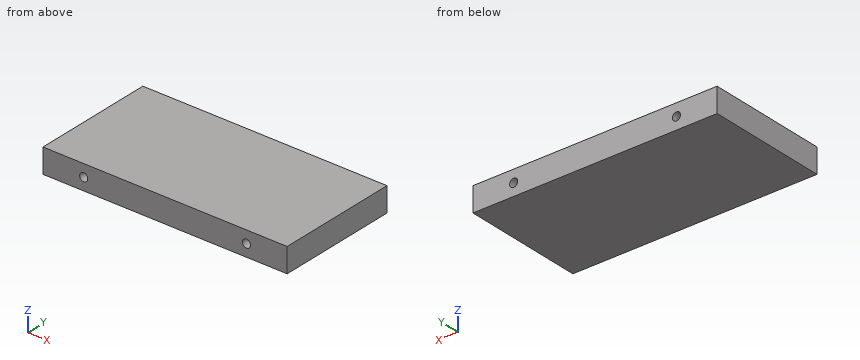
Autodesk Inventor part; units mm, degrees
ref_plane "YZ Plane" through (0, 0, 0) normal (1, 0, 0) x (0, 1, 0)
ref_plane "XZ Plane" through (0, 0, 0) normal (0, 1, 0) x (-1, 0, 0)
ref_plane "XY Plane" through (0, 0, 0) normal (0, 0, 1) x (1, 0, 0)
sketch "Skizze1" plane through (0, 0, 0) normal (0, 1, 0) x (-1, 0, 0)
  line L0 (0, 0) -> (60, 0)
  line L1 (60, 0) -> (60, -6)
  line L2 (60, -6) -> (0, -6)
  line L3 (0, -6) -> (0, 0)
  dimension "d0" = 60
  dimension "d1" = 6
extrude "Extrusion1" add sketch "Skizze1" along normal blind 30
sketch "m" plane through (0, 0, 0) normal (0, -1, 0) x (1, 0, 0)
  line L0 (0, -6) -> (0, 0)
  line L1 (-60, -6) -> (0, -6)
  point P0 (-10, -3)
  point P1 (-50, -3)
  dimension "d4" = 40
  dimension "d5" = 10
  dimension "d6" = 3
hole "Bohrung1" at (-10, 0, -3) at (-50, 0, -3) direction (0, 1, 0) diameter 2 depth 10 tip angle 118
sketch "Skizze3" plane through (0, 30, 0) normal (0, 1, 0) x (1, 0, 0)
  point P0 (0, 0)
  point P1 (-10, 3)
  point P2 (-50, 3)
hole "Bohrung2" at (-10, 30, -3) at (-50, 30, -3) direction (0, -1, 0) diameter 2 depth 10 tip angle 118
properties part number "AkkuHaltSeitenWand"
Geometry: final body of the model. Coordinates: model frame, mm. Give positions to 0.01 mm unless a question says otherwise; leave off trailing zeros. Loops run counter-clockwise (first coordinate to the right, second up) from the corner with the lowest first, then second, coordinate; pieces in that order, holes last. Notation, with made-up numbers: M 23,19 L 57,19 A9 ccw 57,34 Z; hole C 26,41 d6. An arc over 180 degrees is marked long. Put each result on its own line as item: value. Start each with the question number.
1) Cut plane A-A (y = 5.25). Output: boundary loops of the cut face in (x, z), then the cut area to 3 significant figures.
2) Contact query for flat-ended pins moving along their axis: pin 1 (1.2 mm diameter, centred on x = -10, z = -3, fed in from +Y); pin 2 (1.5 mm diameter, centred on x = -26.5, z = -5, fed in from -Y); pin 3 (1.8 mm diameter, centred on x = -10, z = -3, fed in from +Y). Output: stop coordinate, or through.
3) Ray query, line 1 along X through (y, z) = (4.25, -3); line 2 along Z through (x, y) = (-10, 26.5). Return the intervals inside material, ascending.
Verdict:
1. outline: M -60,-6 L 0,-6 L 0,0 L -60,0 Z; hole C -50,-3 d2; hole C -10,-3 d2
1. area: 354 mm2
2. pin 1: y = 19.76
2. pin 2: y = 0
2. pin 3: y = 19.94
3. line 1: -60 to -51, -49 to -11, -9 to 0
3. line 2: -6 to -4, -2 to 0
